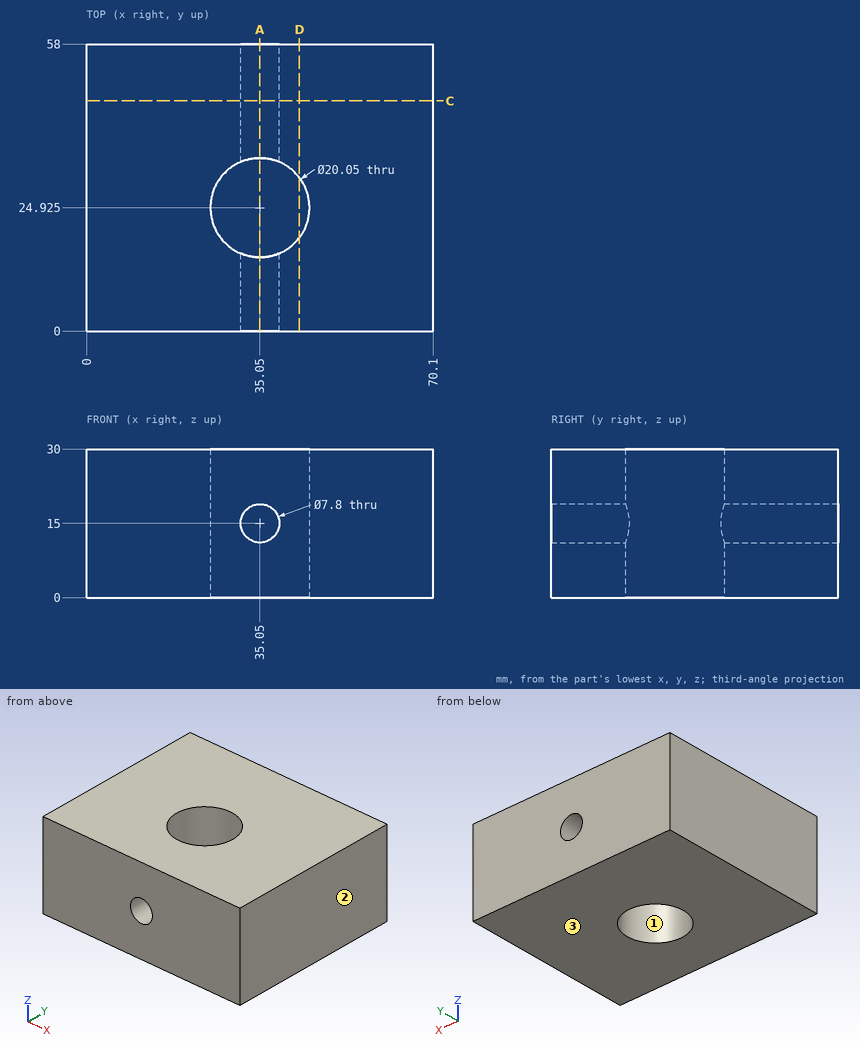
Check sheet for the drawn part. Datum: minimum x, y, z corner. Units: mm. Give positions to 0.01 mm unless a question says otherwise; leave off trailing zeros. Order: outer loops, then holes, each group sorted by start corner. A loop starts at its lowest first (then second) coordinate and runs counter-clockwise, first axis right, second up. Notation, with made-up numbers: (54, 87.25) - (112, 87.25) arc R14 ccw to (112, 113.25) - close; hole circle Ø1 at (-7.75, -24.5). An arc over 180 degrees is marked (long way). Answer in a Markdown table with one row per item. Add a question column.
Q1. Mould release check, pull along X, two halves, no side actions. Record for the marked faces 1, 2 and 3: pulls with the +X half, pulls with the -X half, needs draft (parallel to the pull), parting line crosses it, or undercut.
Q2. Cross-section at A-A, the plane x = 35.05. Enter the section's corners in (y, z).
Q3. Cross-section at D-D, the plane x = 43. Enter the section's corners in (y, z), then the cut area to 3 significant figures.
Q4. Cross-section at C-C, the plane y = 46.5. Enter the section's corners in (x, z), then the cut area to 3 significant figures.
Q5. Material ranges on probe 1 along Z at (x, y) = (35.05, 49.25); probe 2 along Y at (x, z) = (31, 2.5) (1 decimal); probe 3 along Y at (x, z) = (35.05, 9), recorded low to high. Write a range as from..to.
Check values:
| question | item | result |
|---|---|---|
| 1 | face 1 | undercut |
| 1 | face 2 | pulls with the +X half |
| 1 | face 3 | needs draft |
| 2 | outline | (0, 0) - (14.9, 0) - (14.9, 11.1) - (0, 11.1) - close; (0, 18.9) - (14.9, 18.9) - (14.9, 30) - (0, 30) - close; (34.95, 0) - (58, 0) - (58, 11.1) - (34.95, 11.1) - close; (34.95, 18.9) - (58, 18.9) - (58, 30) - (34.95, 30) - close |
| 3 | outline | (0, 0) - (18.82, 0) - (18.82, 30) - (0, 30) - close; (31.03, 0) - (58, 0) - (58, 30) - (31.03, 30) - close |
| 3 | area | 1,370 mm^2 |
| 4 | outline | (0, 0) - (70.1, 0) - (70.1, 30) - (0, 30) - close; hole circle Ø7.8 at (35.05, 15) |
| 4 | area | 2,060 mm^2 |
| 5 | probe 1 | z = 0..11.1, 18.9..30 |
| 5 | probe 2 | y = 0..15.8, 34.1..58 |
| 5 | probe 3 | y = 0..14.9, 34.95..58 |
